```python
from build123d import *

# Parameters (mm, degrees)
F0_R     = 60
F1_DEPTH = 25
F2_SIZE2 = 7.5
F2_SIZE  = 10
F3_SIZE2 = 14.99999
F3_SIZE  = 19.99999


# Not quite as in the source:
# - a fillet or chamfer is up to 0.001 mm smaller than in the source, because OpenCascade refuses the exact size


with BuildPart() as f1:
    # F0 (on Front) → F1 (new body)
    with BuildSketch(Plane.XZ):
        Circle(F0_R)
        with BuildLine():
            ThreePointArc((5.9278272092, 13.7790008556), (12.5283160907, 8.2487148048), (15, 0))
            ThreePointArc((15, 0), (-8.2487148048, -12.5283160907), (-5.9278272092, 13.7790008556))
            Line((-5.9278272092, 13.7790008556), (-5.9278272092, 20.3793700784))
            Line((-5.9278272092, 20.3793700784), (5.9278272092, 20.3793700784))
            Line((5.9278272092, 20.3793700784), (5.9278272092, 13.7790008556))
        make_face(mode=Mode.SUBTRACT)
    extrude(amount=F1_DEPTH)

    # F2
    f2_edges = [f1.edges().sort_by_distance(p)[0] for p in [
        (-60, 0, 0),
    ]]
    f2_side = f1.faces().sort_by_distance((-60, -12.5, 0))[0]
    chamfer(f2_edges, length=F2_SIZE, length2=F2_SIZE2, reference=f2_side)

    # F3 (size 20 and 15 in the source; OpenCascade refuses exactly that, so slightly less here)
    f3_edges = [f1.edges().sort_by_distance(p)[0] for p in [
        (-60, -25, 0),
    ]]
    f3_side = f1.faces().sort_by_distance((-58.302944, -25, 0))[0]
    chamfer(f3_edges, length=F3_SIZE, length2=F3_SIZE2, reference=f3_side)


solid = f1.part
```
Input: part model. Units: mm. Frame: model coordinates. A direction names the side the tool comes from. Coordinates: 2 decimals unless noted, no trailing zeros. Loops run counter-clockwise (first coordinate to the right, second up) from the corner with the lowest first, then second, coordinate; pieces in that order, holes last. Notation, with made-up numbers: M 11,65 L 31,65 A30 cw 31,95 Z; hole C 34,17.25 d2. An arc over 180 degrees is marked long. One line per item, written item: value.
(1) Reachability of faces 4 (the flat face through (-1, -25, -17)), 5 (the flat face through (0, -12, 20.379)) from +Z, -Z, +X, -X, +Y, -Y: full face, straight path, thin tool, end or side. Return the list, or none.
Filled in:
face 4: +Z, -Z, +X, -X, -Y
face 5: +Y, -Y
(2) Pull-direction query (X, two-part tool) for faces 1 (the conical face through (-8.94, -24.06, -40.27)), 2 (the flat face through (11, 0, -11)), 3 (the flat face through (5.928, -12, 17)); classes: +X half, -X half, draft (parallel to the pull), parting line (faces both ways), or undercut.
Filled in:
face 1: parting line
face 2: draft
face 3: undercut
(3) Line query: line 1 along Z through (x, y) = (0, -13.25); line 2 along Z through (x, y) = (4, -23); line 3 along X through (y, z) = (-1.5, 29.5). Output: solid intervals per line, ascending. Write a range as from..to.
Filled in:
line 1: -55.67..-15, 20.38..55.67
line 2: -42.48..-14.46, 20.38..42.48
line 3: -44.78..44.78
(4) Pin query (flat end, axial travel): pin 1 (1.5 mm diameter, centred on x = -16.5, y = -6.5, fed in from -Z); pin 2 (2 mm diameter, centred on x = -21, y = -19.5, fed in from +Z); pin 3 (2 mm diameter, centred on y = -11.5, z = 15.5, fed in from -X). Return the tip coordinate at first contact, or that it passes through.
Filled in:
pin 1: z = -55.58
pin 2: z = 43.98
pin 3: x = -57.3
(5) Section B-B (y = -3.75). Output: boundary loops of the cut face in (x, z) (1 decimal), and give its area (3 significant figures).
Filled in:
outline: C 0,0 d110.6; hole M -5.9,13.8 A15 ccw long 5.9,13.8 L 5.9,20.4 L -5.9,20.4 Z
area: 8,840 mm^2
(6) Section C-C (y = -22.75). Output: boundary loops of the cut face in (x, z).
Filled in:
outline: C 0,0 d86; hole M -5.93,13.78 A15 ccw long 5.93,13.78 L 5.93,20.38 L -5.93,20.38 Z
